```python
from build123d import *

# Parameters (mm, degrees)
MODEL_R                 = 1.5
SALIENTE_EXTRUIR1_DEPTH = 3


with BuildPart() as part:
    # Model → Saliente-Extruir1 (new body)
    with BuildSketch(Plane.XY):
        with BuildLine():
            Line((47.956564936, 294.416156902), (47.956564936, 276.316156902))
            ThreePointArc((47.956564936, 276.316156902), (48.482384187, 274.205259611), (49.936959325, 272.587673623))
            Line((49.936959325, 272.587673623), (70.456564936, 258.72109315))
            Line((70.456564936, 258.72109315), (79.456564936, 252.639142716))
            Line((79.456564936, 252.639142716), (79.456564936, 249.316156902))
            ThreePointArc((79.456564936, 249.316156902), (83.956564936, 244.816156902), (88.456564936, 249.316156902))
            Line((88.456564936, 249.316156902), (88.456564456, 249.318235809))
            Line((88.456564456, 249.318235809), (88.454517382, 258.180422621))
            ThreePointArc((88.454517382, 258.180422621), (88.187667044, 259.848401972), (87.32462533, 261.300477459))
            Line((87.32462533, 261.300477459), (65.956564936, 285.416156902))
            Line((65.956564936, 285.416156902), (65.956564936, 294.316156902))
            ThreePointArc((65.956564936, 294.316156902), (64.638545451, 297.498137417), (61.456564936, 298.816156902))
            Line((61.456564936, 298.816156902), (52.356564936, 298.816156902))
            ThreePointArc((52.356564936, 298.816156902), (49.245295099, 297.527426739), (47.956564936, 294.416156902))
        make_face()
        with Locations((83.956564936, 249.316156902)):
            Circle(MODEL_R, mode=Mode.SUBTRACT)
        with Locations((70.456564936, 267.316156902)):
            Circle(MODEL_R, mode=Mode.SUBTRACT)
        with Locations((83.956564936, 258.316156902)):
            Circle(MODEL_R, mode=Mode.SUBTRACT)
        with Locations((52.456564936, 276.316156902)):
            Circle(MODEL_R, mode=Mode.SUBTRACT)
        with Locations((61.456564936, 276.316156902)):
            Circle(MODEL_R, mode=Mode.SUBTRACT)
        with Locations((52.456564936, 285.316156902)):
            Circle(MODEL_R, mode=Mode.SUBTRACT)
        with Locations((52.456564936, 294.316156902)):
            Circle(MODEL_R, mode=Mode.SUBTRACT)
        with Locations((61.456564936, 285.316156902)):
            Circle(MODEL_R, mode=Mode.SUBTRACT)
        with Locations((61.456564936, 294.316156902)):
            Circle(MODEL_R, mode=Mode.SUBTRACT)
    extrude(amount=SALIENTE_EXTRUIR1_DEPTH)


solid = part.part
```
CAD build for the part. Positions are in the model's coordinates, mm. A direction names the side the tool comes from. Round coordinates to 2 decimals unless told otherwise and drop trailing zeros. Loops run counter-clockwise (first coordinate to the right, second up) from the corner with the lowest first, then second, coordinate; pieces in that order, holes last. Notation, with made-up numbers: (38, 36) - (90, 36) arc R12 cw to (90, 57) - close; hole circle Ø3 at (73.5, 23). An arc over 180 degrees is marked (long way). Return JSON: item names as keys, results as strings. Group by question number.
Q1. Two-plate mould, pull along X, no slides. Class faces 1 (the face through (53.263, 295.581, 1.479)), 2 (the face through (68, 272, 0)), 3 (the face through (88.196, 259.826, 1.479)): +X half, -X half, draft (parallel to the pull), parting line (faces both ways), or undercut.
Q2. Band-saw the part on B-B on y = 290. Give the cut face in (x, z), plus the area to 3 significant figures.
Q3. Band-saw the part on C-C on x = 81.5. Give the cut face in (y, z).
Q4. Flat gauge pins, fed straight in: pin 1 Ø2.5 at (x, y) = (52.46, 294.32) entering from +Z; pin 2 Ø1 at (y, z) = (262.5, 2) entering from +X; pin 3 Ø1 at (y, z) = (262, 2) entering from -X; pin 4 Ø0.9 at (y, z) = (251, 2) entering from -X. Where does each tip first touch, or does it go through?
Q5. Tool access for faces 4 (the face through (79.457, 251, 1)), 5 (the face through (65.957, 290, 1)), 6 (the face through (57, 298.816, 1)): list every direction of +Z, -Z, +X, -X, +Y, -Y with a clear straight run to the whole face (end or side of a thin tool).
Q6. Drill centre lines: line 1 along Y through (x, z) = (60.5, 2.3); line 2 along Y through (x, z) = (51.5, 1.05); line 3 along X through (y, z) = (289, 2.7). Where is each one in solid material? Low to high. Write a range as [from, to].
Q7. Band-saw the part on A-A on z = 0.6. Give the number of separate pieces and of enclosed holes in the cut face, plus the area to 3 significant figures.
Solutions:
{
 "1": {"face 1": "undercut", "face 2": "draft", "face 3": "+X half"},
 "2": {"outline": "(47.96, 0) - (65.96, 0) - (65.96, 3) - (47.96, 3) - close", "area": "54.0 mm^2"},
 "3": {"outline": "(245.55, 0) - (267.87, 0) - (267.87, 3) - (245.55, 3) - close"},
 "4": {"pin 1": "passes through", "pin 2": "stops at x = 86.7", "pin 3": "stops at x = 64.86", "pin 4": "stops at x = 79.46"},
 "5": {"face 4": "+Z, -Z, -X, -Y", "face 5": "+Z, -Z, +X, +Y", "face 6": "+Z, -Z, +X, -X, +Y"},
 "6": {"line 1": "y = [265.45, 275.16], [277.47, 284.16], [286.47, 293.16], [295.47, 298.82]", "line 2": "y = [271.53, 275.16], [277.47, 284.16], [286.47, 293.16], [295.47, 298.73]", "line 3": "x = [47.96, 65.96]"},
 "7": {"separate pieces": "1", "enclosed holes": "9", "area": "936 mm^2"}
}
